The model under review builds one solid part; all positions refer to its coordinate system, in mm. A direction names the side the tool comes from. Round coordinates to 2 decimals unless told otherwise and drop trailing zeros. Order: outer loops, then holes, each group sorted by start corner. A loop starts at its lowest first (then second) coordinate and runs counter-clockwise, first axis right, second up. Notation, with made-up numbers: (70.25, -11) -> (87.25, -11) arc R25 ccw to (87.25, 27) -> close; hole circle Ø6 at (82.25, 63.5). An arc over 180 degrees is marked (long way). Use a Markdown table: item, result. Add a question column.
```python
from build123d import *

# Parameters (mm, degrees)
SKETCH1_R           = 4
BOSS_EXTRUDE1_DEPTH = 2.3
SKETCH2_R           = 2
BOSS_EXTRUDE2_DEPTH = 9.7
CHAMFER1_SIZE       = 0.3
CUT_EXTRUDE1_DEPTH  = 2
CHAMFER2_SIZE       = 2.4


with BuildPart() as part:
    # Sketch1 → Boss-Extrude1 (new body)
    with BuildSketch(Plane.XY):
        Circle(SKETCH1_R)
    extrude(amount=BOSS_EXTRUDE1_DEPTH)

    # Sketch2 → Boss-Extrude2 (add)
    with BuildSketch(Plane(origin=(0, 0, 0), x_dir=(-1, 0, 0), z_dir=(0, 0, -1))):
        with Locations(Location((0, 0, 0), (0, 0, 180))):
            Circle(SKETCH2_R)
    extrude(amount=BOSS_EXTRUDE2_DEPTH)

    # Chamfer1
    chamfer1_edges = [part.edges().sort_by_distance(p)[0] for p in [
        (-2, 0, -9.7),
    ]]
    chamfer(chamfer1_edges, length=CHAMFER1_SIZE)

    # Sketch3 → Cut-Extrude1 (cut)
    with BuildSketch(Plane.XY.offset(2.3)):
        Polygon((0, 1.443375673), (-1.25, 0.721687836), (-1.25, -0.721687836), (0, -1.443375673), (1.25, -0.721687836), (1.25, 0.721687836), align=None)
    extrude(amount=-CUT_EXTRUDE1_DEPTH, mode=Mode.SUBTRACT)

    # Chamfer2
    # the kernel refuses this chamfer: 2.4 mm, written as the material it takes off along each edge
    with BuildSketch(Plane(origin=(0, 0, 0), x_dir=(1, 0, 0), z_dir=(0, -1, 0))) as chamfer2_piece_1_section:
        Polygon((4 - CHAMFER2_SIZE, 0), (4, CHAMFER2_SIZE), (4, 0), align=None)
    chamfer2_piece_1 = revolve(axis=Axis((0, 0, 0), (0, 0, 1)), mode=Mode.PRIVATE)
    chamfer2_piece_1 = chamfer2_piece_1 - Plane(origin=(0, 0, 1.405884102), x_dir=(1, 0, 0), z_dir=(0, 0, 1)) * Cylinder(2, 16, mode=Mode.PRIVATE)
    add(chamfer2_piece_1, mode=Mode.SUBTRACT)


solid = part.part
```
Q1. Wall thickness on line 1 (Y direction, x = 1, z = 1.25); line 2 (X direction, y = -0.25, z = 1.75); line 3 (Y direction, x = -0.5, z = -5.25): over which ranges is each line inside the solid? List them lowest first. Write a range as [from, to].
Q2. Add section A-A (z = 1). Write out the cut boundary in (x, y).
Q3. Add section B-B (y = 0). Write out the cut boundary in (x, z), then the cut area to 3 significant figures.
Q4. Mouldability with a two-part tool opening along Y and no side actions: class faces 3 (the flat face through (2, 0, 2.3)), 4 (the conical face through (2.02, 0.64, 0.52)), 5 (the flat face through (-1.25, 0, 1)) as pulls with the +Y half, pulls with the -Y half, needs draft (parallel to the pull), parting line crosses it, or undercut.
Q5. Add section C-C (z = -5.5). Write out the cut boundary in (x, y), then the cut area to 3 significant figures.
Q6. Insertion check: pin 1 (1.5 mm diameter, centred on y = 0, z = -2.5, fed in from +X); pin 2 (0.7 mm diameter, centred on y = -0.5, z = 1.5, fed in from +X); pin 3 (1 mm diameter, centred on x = 1, z = -7, fed in from +Y); pin 4 (2 mm diameter, centred on x = 0.5, y = -0.5, fed in from +Z). Each pin has a flat end and moves straight along its axis. Give the tip position at first contact, or say it passes through.
Q7. Machinability: for faces 1 (the flat face through (1.25, 0, 1)), 2 (the flat face through (0, 0, -9.7)), which of the approach directions +Z, -Z, +X, -X, +Y, -Y give a long, thin tool a straight path to every point of the face, cutting with its end or side? Answer none if there is none.
Report:
| question | item | result |
|---|---|---|
| 1 | line 1 | y = [-2.67, -0.87], [0.87, 2.67] |
| 1 | line 2 | x = [-3.34, -1.25], [1.25, 3.34] |
| 1 | line 3 | y = [-1.94, 1.94] |
| 2 | outline | circle Ø5.2 at (0, 0); hole (-1.25, -0.72) -> (0, -1.44) -> (1.25, -0.72) -> (1.25, 0.72) -> (0, 1.44) -> (-1.25, 0.72) -> close |
| 3 | outline | (-3.9, 2.3) -> (-2, 0.4) -> (-2, -9.4) -> (-1.7, -9.7) -> (1.7, -9.7) -> (2, -9.4) -> (2, 0.4) -> (3.9, 2.3) -> (1.25, 2.3) -> (1.25, 0.3) -> (-1.25, 0.3) -> (-1.25, 2.3) -> close |
| 3 | area | 46.5 mm² |
| 4 | face 3 | needs draft |
| 4 | face 4 | parting line crosses it |
| 4 | face 5 | undercut |
| 5 | outline | circle Ø4 at (0, 0) |
| 5 | area | 12.6 mm² |
| 6 | pin 1 | stops at x = 2 |
| 6 | pin 2 | stops at x = 3.42 |
| 6 | pin 3 | stops at y = 1.94 |
| 6 | pin 4 | stops at z = 2.3 |
| 7 | face 1 | +Z |
| 7 | face 2 | -Z, +X, -X, +Y, -Y |
